Here's how the part is built. I have some questions about the finished solid (model axes, mm). Coordinates: 2 decimals unless noted, no trailing zeros. Order: outer loops, then holes, each group sorted by start corner. A loop starts at its lowest first (then second) coordinate and runs counter-clockwise, first axis right, second up. Notation, with made-up numbers: M -0.5,85 L 46.5,85 A18 cw 46.5,92 Z; hole C 2,-34.75 d8. An arc over 180 degrees is marked long. Answer as CSV lines item,"result". Start each with the question number.
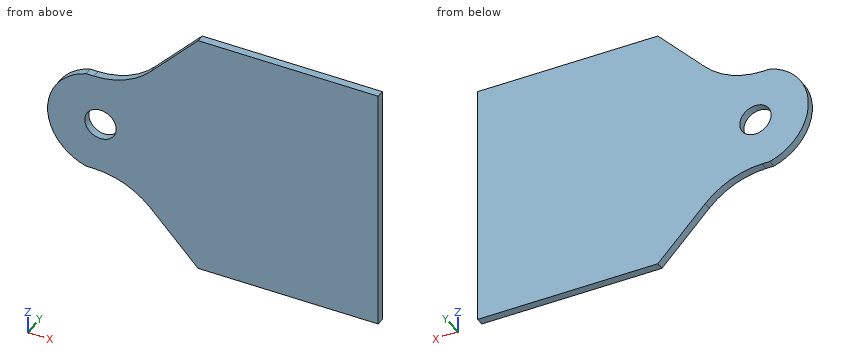
```python
from build123d import *

# Parameters (mm, degrees)
SKETCH_1_R      = 4
EXTRUDE_1_DEPTH = 2


with BuildPart() as part:
    # 草图1 → 凸台-拉伸1 (new body)
    with BuildSketch(Plane(origin=(0, 0, 0), x_dir=(1, 0, 0), z_dir=(0, 1, 0))):
        with BuildLine():
            Line((-49.618188819, -13), (-51.618188819, -13))
            ThreePointArc((-51.618188819, -13), (-61.441082992, 0), (-51.618188819, 13))
            Line((-51.618188819, 13), (-49.618188819, 13))
            ThreePointArc((-49.618188819, 13), (-41.703538748, 14.632683531), (-35.08110056, 19.264168574))
            Line((-35.08110056, 19.264168574), (-23, 32.05))
            Line((-23, 32.05), (23, 32.05))
            Line((23, 32.05), (23, -32.05))
            Line((23, -32.05), (-23, -32.05))
            Line((-23, -32.05), (-35.08110056, -19.264168574))
            ThreePointArc((-35.08110056, -19.264168574), (-41.703538748, -14.632683531), (-49.618188819, -13))
        make_face()
        with Locations((-47.927283228, 0)):
            Circle(SKETCH_1_R, mode=Mode.SUBTRACT)
    extrude(amount=EXTRUDE_1_DEPTH)


solid = part.part
```
1) Suppose I cut it at D-D on z = -9.5. Please give me the cut outline in (x, y), plus the area to 3 significant figures.
2) Suppose I cut it at A-A on z = 0. Please give me the cut outline in (x, y).
3) Suppose I cut it at B-B on y = 1.3. Please give me the cut outline in (x, z), plus the area to 3 significant figures.
4) I need wall thicknesses on line 1 (X direction, y = 1.4, z = 0); line 2 (Z direction, x = -29, y = 1.1); line 3 (Z direction, x = -36, y = 1.4). Which ranges of each line are inside material? Lowest first, please. Write a range as [from, to].
5) Suppose I cut it at C-C on x = -33.5. Please give me the cut outline in (y, z), plus the area to 4 significant figures.
6) Will this pin go through, and if not, where does the flat tip stop? pin 1 Ø1 at (x, y) = (-50.5, 1) entering from -Z.
Output:
1,outline,"M -57.54,0 L 23,0 L 23,2 L -57.54,2 Z"
1,area,"161 mm²"
2,outline,"M -61.44,0 L -51.93,0 L -51.93,2 L -61.44,2 Z; M -43.93,0 L 23,0 L 23,2 L -43.93,2 Z"
3,outline,"M -51.62,-13 L -49.62,-13 A20 cw -35.08,-19.26 L -23,-32.05 L 23,-32.05 L 23,32.05 L -23,32.05 L -35.08,19.26 A20 cw -49.62,13 L -51.62,13 A13.51 ccw Z; hole C -47.93,0 d8"
3,area,"4,190 mm²"
4,line 1,"[-61.44, -51.93], [-43.93, 23]"
4,line 2,"[-25.7, 25.7]"
4,line 3,"[-18.35, 18.35]"
5,outline,"M 0,-20.94 L 2,-20.94 L 2,20.94 L 0,20.94 Z"
5,area,"83.75 mm²"
6,pin 1,"z = -13"
